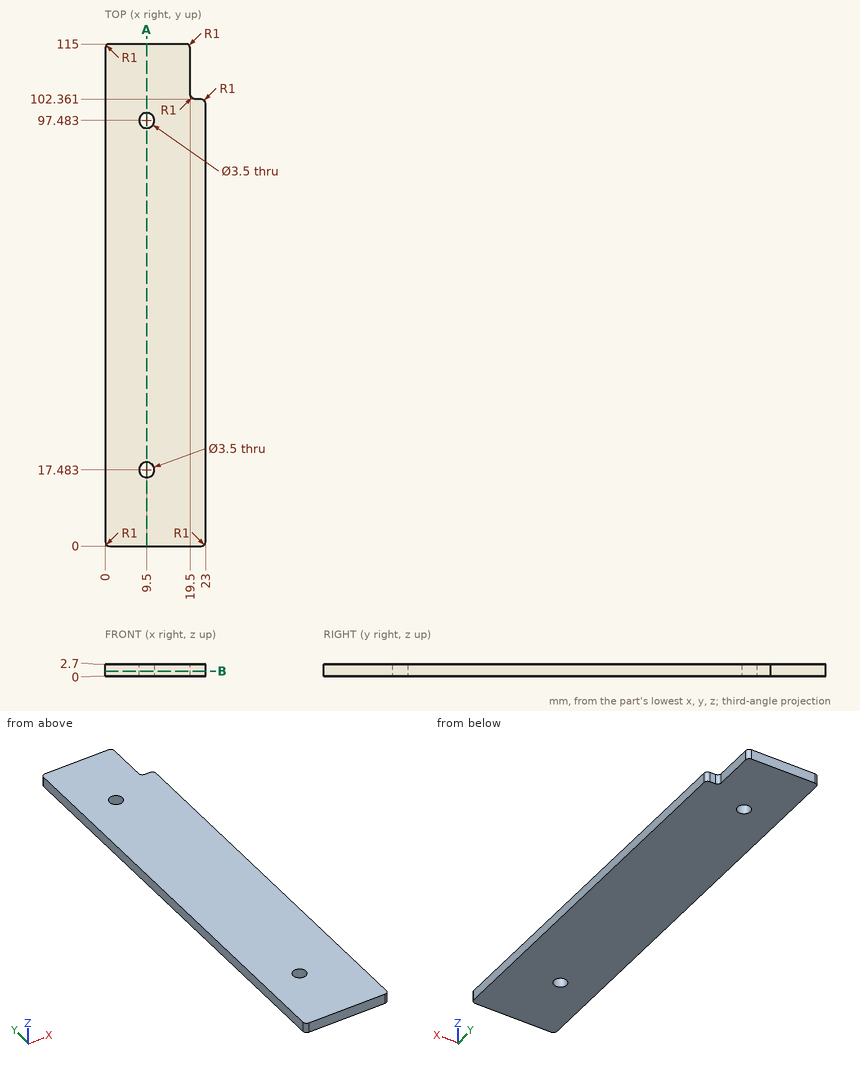
Job drawing, mm, ordinate dimensions from the low corner. One solid piece. Round coordinates to 2 decimals unless told otherwise and drop trailing zeros. Loops run counter-clockwise (first coordinate to the right, second up) from the corner with the lowest first, then second, coordinate; pieces in that order, holes last. Notation, with made-up numbers: (5.25, 2.5) -> (22.25, 2.5) arc R18 cw to (22.25, 8.5) -> close; hole circle Ø1 at (-5, 36). An arc over 180 degrees is marked (long way). Use a Markdown table: item, result.
1) Drop a flat-ended pin along its axis: pin 1 Ø1.2 at (x, z) = (21.5, 1.5) entering from +Y. Give the stop position or say it passes through.
The answers:
| item | result |
|---|---|
| pin 1 | stops at y = 102.36 |
2) Cut at B-B, the plane z = 1.1. List the corners of the cut face in (x, y), and give its area (3 significant figures).
The answers:
| item | result |
|---|---|
| outline | (0, 1) arc R1 ccw to (1, 0) -> (22, 0) arc R1 ccw to (23, 1) -> (23, 101.36) arc R1 ccw to (22, 102.36) -> (20.5, 102.36) arc R1 cw to (19.5, 103.36) -> (19.5, 114) arc R1 ccw to (18.5, 115) -> (1, 115) arc R1 ccw to (0, 114) -> close; hole circle Ø3.5 at (9.5, 17.48); hole circle Ø3.5 at (9.5, 97.48) |
| area | 2,580 mm2 |
3) Cut at A-A, the plane x = 9.5. List the corners of the cut face in (y, z).
The answers:
| item | result |
|---|---|
| outline | (0, 0) -> (15.73, 0) -> (15.73, 2.7) -> (0, 2.7) -> close; (19.23, 0) -> (95.73, 0) -> (95.73, 2.7) -> (19.23, 2.7) -> close; (99.23, 0) -> (115, 0) -> (115, 2.7) -> (99.23, 2.7) -> close |
4) Probe line 1 (Y direction, x = 9.5, z = 2.05); line 2 (Y direction, x = 8.5, z = 0.85); line 3 (X direction, y = 19, z = 0.7) (1 decimal). List the from-to ranges inside material, lowest first. Write a range as [from, to].
The answers:
| item | result |
|---|---|
| line 1 | y = [0, 15.73], [19.23, 95.73], [99.23, 115] |
| line 2 | y = [0, 16.05], [18.92, 96.05], [98.92, 115] |
| line 3 | x = [0, 8.6], [10.4, 23] |
